```python
from build123d import *

# Parameters (mm, degrees)
SKETCH1_W           = 215.9
SKETCH1_H           = 381
BOSS_EXTRUDE1_DEPTH = 6.35
SKETCH2_R           = 190.5
CUT_EXTRUDE1_DEPTH  = 245.802296865
CUT_EXTRUDE2_DEPTH  = 245.802296865


with BuildPart() as part:
    # Sketch1 → Boss-Extrude1 (new body)
    with BuildSketch(Plane(origin=(0, 0, 0), x_dir=(0, 0, -1), z_dir=(1, 0, 0))):
        with Locations((12.7, 22.411764706)):
            Rectangle(SKETCH1_W, SKETCH1_H)
    extrude(amount=BOSS_EXTRUDE1_DEPTH)

    # Sketch2 → Cut-Extrude1 (cut, through all)
    with BuildSketch(Plane(origin=(6.35, 0, 0), x_dir=(0, 0, -1), z_dir=(1, 0, 0))):
        with Locations((-95.25, 22.411764706)):
            Circle(SKETCH2_R)
    extrude(amount=-CUT_EXTRUDE1_DEPTH, mode=Mode.SUBTRACT)

    # Sketch3 → Cut-Extrude2 (cut, through all)
    with BuildSketch(Plane(origin=(6.35, 0, 0), x_dir=(0, 0, -1), z_dir=(1, 0, 0))):
        Polygon((60.798464437, 131.678075831), (-18.968243734, 245.59674111), (-203.446235094, 245.59674111), (-203.446235094, 131.678075831), align=None)
    extrude(amount=-CUT_EXTRUDE2_DEPTH, mode=Mode.SUBTRACT)


solid = part.part
```
CAD build for the part. Positions are in the model's coordinates, mm. Round coordinates to 2 decimals unless told otherwise and drop trailing zeros. Loops run counter-clockwise (first coordinate to the right, second up) from the corner with the lowest first, then second, coordinate; pieces in that order, holes last. Notation, with made-up numbers: M 86,63 L 120,63 A6 cw 120,68 Z; hole C -39.5,79.25 d2. An arc over 180 degrees is marked long. Use a Markdown table: item, result. Add a question column.
(1) Cut at C-C (y = 77.5). Give the cut face in (x, z), and give its area (3 significant figures).
(2) Flat gauge pins, fed straight in: pin 1 (1.5 mm diameter, centred on x = 1, y = 77, fed in from +Z); pin 2 (1.5 mm diameter, centred on x = 2, z = 41, fed in from +Y). Where does each tip first touch, or does it go through?
(3) Pull direction Y, two halves, no side cores. Call faces 1 (the face through (6.35, 9, -100)), 2 (the face through (3.219, 171.726, -32.756)): +Y half, -Y half, draft (parallel to the pull), parting line (faces both ways), or undercut.
(4) Drill centre lines: line 1 (Y direction, x = 4.75, z = -58.5); line 2 (Z direction, x = 2.25, y = 183.5); line 3 (Z direction, x = 4.5, y = 9). Where is each one in solid material? Low to high.
(5) Cut at A-A (z = -74.5). Give the cut face in (x, y).
(6) Cut at B-B (x = 3.5). Give the cut face in (y, z).
Geometry says:
| question | item | result |
|---|---|---|
| 1 | outline | M 0,-120.65 L 6.35,-120.65 L 6.35,-87.11 L 0,-87.11 Z |
| 1 | area | 213 mm² |
| 2 | pin 1 | stops at z = -87.04 |
| 2 | pin 2 | stops at y = -159.98 |
| 3 | face 1 | draft |
| 3 | face 2 | undercut |
| 4 | line 1 | y = -168.09 to -90.07, 134.96 to 212.91 |
| 4 | line 2 | z = -120.65 to -24.51 |
| 4 | line 3 | z = -120.65 to -94.78 |
| 5 | outline | M 0,-168.09 L 6.35,-168.09 L 6.35,-64.05 L 0,-64.05 Z; M 0,108.87 L 6.35,108.87 L 6.35,212.91 L 0,212.91 Z |
| 6 | outline | M -168.09,-120.65 L 212.91,-120.65 L 212.91,-3.92 L 131.68,-60.8 A190.5 cw -168.09,95.25 Z |
